from build123d import *

# Parameters (mm, degrees)
SKETCH003_W   = 322
SKETCH003_H   = 270
SKETCH003_R   = 97
SKETCH003_R_2 = 9
PAD003_DEPTH  = 34
PAD004_DEPTH  = 180
SKETCH005_R   = 9
HOLE_DEPTH    = 34


with BuildPart() as part:
    # Sketch003 (on Face1 of ShapeBinder) → Pad003 (new body)
    with BuildSketch(Plane(origin=(0, 0, 0), x_dir=(1, 0, 0), z_dir=(0, 0, -1))):
        with Locations((-0.5, 0)):
            Rectangle(SKETCH003_W, SKETCH003_H)
        Circle(SKETCH003_R, mode=Mode.SUBTRACT)
        with Locations((-125.5, 100.5)):
            Circle(SKETCH003_R_2, mode=Mode.SUBTRACT)
        with Locations((125.5, 100.5)):
            Circle(SKETCH003_R_2, mode=Mode.SUBTRACT)
        with Locations((-125.5, -100.5)):
            Circle(SKETCH003_R_2, mode=Mode.SUBTRACT)
        with Locations((125.5, -100.5)):
            Circle(SKETCH003_R_2, mode=Mode.SUBTRACT)
    extrude(amount=PAD003_DEPTH)

    # Sketch004 (on Face1 of Pad003) → Pad004 (join)
    with BuildSketch(Plane.XZ.offset(135)):
        Polygon((-161.5, -34), (-122.75, -34), (-103.120091, -68), (-161.5, -68), align=None)
    pad004 = extrude(amount=-PAD004_DEPTH)

    # Mirrored: Pad004 across Sketch004 V_Axis
    add(pad004.mirror(Plane(origin=(0, -135, 0), x_dir=(0, -1, 0), z_dir=(1, 0, 0))))

    # Sketch005 (on Face6 of Mirrored) → Hole (cut)
    with BuildSketch(Plane(origin=(0, 0, -34), x_dir=(1, 0, 0), z_dir=(0, 0, -1))):
        with Locations((-112.935045, 60)):
            Circle(SKETCH005_R)
        with Locations((-112.935045, -60)):
            Circle(SKETCH005_R)
        with Locations((112.935045, 60)):
            Circle(SKETCH005_R)
        with Locations((112.935045, -60)):
            Circle(SKETCH005_R)
    extrude(amount=-HOLE_DEPTH, mode=Mode.SUBTRACT)


solid = part.part
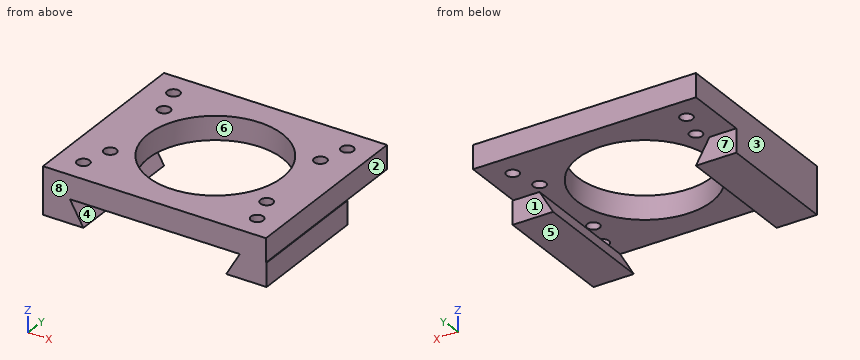
Check sheet for the modelled part. Datum: model origin and axes. Units: mm. Face numbers are marked on the shaded views. A direction names the side the tool comes from. Give positions to 0.01 mm unless a question says otherwise; leave off trailing zeros. Write each loop counter-clockwise with the first axis right and the second up, starting at its lowest first coordinate (ties: lowest second). Pieces come first, ordered by that corner, then holes. Notation, with made-up numbers: (-40, 67) -> (-8, 67) arc R21 cw to (-8, 85) -> close; hole circle Ø5 at (43, -24.75). An arc over 180 degrees is marked (long way). Write item = value, one per line.
Item 1: Sectioned sample at C-C on z = -13.5. Count the separate pieces of the cut face and the enclosed holes in it, and give its area (3 significant figures).
Output:
separate_pieces = 1
enclosed_holes = 9
area = 55,300 mm^2
Item 2: Scan lines: probe 1 along X at (y, z) = (-100.5, -17); probe 2 along Y at (x, z) = (-125.5, -11.5); probe 3 along Y at (x, z) = (0, -10). Record each from-to range of solid material in increasing order. Write a range as from..to.
Output:
probe_1 = -161.5..-134.5, -116.5..116.5, 134.5..160.5
probe_2 = -135..-109.5, -91.5..91.5, 109.5..135
probe_3 = -135..-97, 97..135
Item 3: Sectioned sample at A-A on y = 0. Record the boundary of the cut face in (x, z).
Output:
outline = (-161.5, -68) -> (-103.12, -68) -> (-122.75, -34) -> (-97, -34) -> (-97, 0) -> (-161.5, 0) -> close; (97, -34) -> (122.75, -34) -> (103.12, -68) -> (161.5, -68) -> (161.5, -34) -> (160.5, -34) -> (160.5, 0) -> (97, 0) -> close
Item 4: Gauge pin test, flat ends, axial feed: pin 1 (13 mm diameter, centred on x = -130, y = -100, fed in from +Z); pin 2 (14.5 mm diameter, centred on x = -125.5, y = 100.5, fed in from +Z); pin 3 (3 mm diameter, centred on x = -88, y = 107, fed in from -Z); pin 4 (3.5 mm diameter, centred on x = 131.5, y = -102, fed in from +Z). Record the tip position at first contact, or that the pin passes through.
Output:
pin_1 = 0
pin_2 = through
pin_3 = -34
pin_4 = -34
Item 5: Sectioned sample at B-B on x = 0. Record the boundary of the cut face in (y, z).
Output:
outline = (-135, -34) -> (-97, -34) -> (-97, 0) -> (-135, 0) -> close; (97, -34) -> (135, -34) -> (135, 0) -> (97, 0) -> close
Item 6: Sectioned sample at D-D on y = 100.5. Record the boundary of the cut face in (x, z).
Output:
outline = (-161.5, -34) -> (-134.5, -34) -> (-134.5, 0) -> (-161.5, 0) -> close; (-116.5, -34) -> (116.5, -34) -> (116.5, 0) -> (-116.5, 0) -> close; (134.5, -34) -> (160.5, -34) -> (160.5, 0) -> (134.5, 0) -> close
Item 7: Tool access check on the marked faces 1, 2, 3 and 4. Record the directions out of +Z, -Z, +X, -X, +Y, -Y that give a thin tool (end or side, any length) a straight path to the whole face; none if there is none.
Output:
face_1 = -Z, +X, -X, +Y
face_2 = +Z, +X, +Y, -Y
face_3 = +Z, -Z, -X, +Y, -Y
face_4 = +Y, -Y
Item 8: Release check for a two-part mould opening along Y. For the marked faces 5, 6, 7 and 8 record: +Y half, -Y half, draft (parallel to the pull), parting line (faces both ways), or undercut.
Output:
face_5 = draft
face_6 = undercut
face_7 = +Y half
face_8 = -Y half
